Could you check a few things on this model? Use its own coordinates, in mm. Give positions to 0.01 mm unless a question says otherwise; leave off trailing zeros. Write each loop counter-clockwise with the first axis right and the second up, starting at its lowest first coordinate (ties: lowest second). Pieces come first, ordered by that corner, then holes. Notation, with made-up numbers: M 78.25,33 L 85.25,33 A27 ccw 85.25,67 Z; hole C -7.75,7.25 d4. An arc over 180 degrees is marked long. Answer as CSV lines item,"result". Start each with the question number.
from build123d import *

# Parameters (mm, degrees)
SKETCH1_W           = 42.637682839
SKETCH1_H           = 10
BOSS_EXTRUDE1_DEPTH = 2


with BuildPart() as part:
    # Sketch1 → Boss-Extrude1 (new body)
    with BuildSketch(Plane.XY):
        Polygon((0, 20), (9.5, 20), (9.5, 5.999528404), (41.549837727, 5.999528404), (41.549837727, 20), (41.549837727, 22), (80.459837727, 22), (80.459837727, 20), (115.41, 20), (115.41, 15), (117.41, 15), (117.41, 5), (115.41, 5), (115.41, 0), (80.459837727, 0), (80.459837727, -2.000471596), (35.049837727, -2.000471596), (35.049837727, 0), (0, 0), (0, 5), (-2, 5), (-2, 15), (0, 15), align=None)
        with Locations((65.091158581, 11)):
            Rectangle(SKETCH1_W, SKETCH1_H, mode=Mode.SUBTRACT)
    extrude(amount=BOSS_EXTRUDE1_DEPTH)


solid = part.part
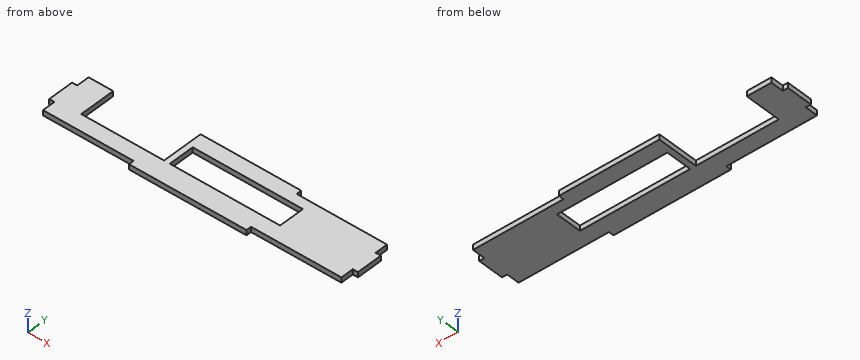
1. Imagine slicing it at B-B, the plane z = 1.1. Please give me the cut outline in (x, y), plus the area to 3 significant figures.
2. Imagine slicing it at A-A, the plane y = 9.5. Please give me the cut outline in (x, z).
3. Imagine slicing it at D-D, the plane y = 18.5. Please give me the cut outline in (x, z).
4. Please list where these lines run through material, in increasing order: line 1 (X direction, y = 11, z = 0.35); line 2 (Y direction, x = 76.5, z = 1.3); line 3 (X direction, y = 16.25, z = 0.6).
5. Imagine slicing it at C-C, the plane x = 75. Please give me the cut outline in (y, z).
6. Will these pins go through, and if not, where does the flat tip stop? P1, Ø1, axis at y = 1, z = 0.5, coming from the +X side; P2, Ø1, axis at x = -1, z = 1, coming from the -Y side; P3, Ø1, axis at x = 101.5, z = 1.5, coming from the +Y side.
Solutions:
1,outline,"M -2,5 L 0,5 L 0,0 L 35.05,0 L 35.05,-2 L 80.46,-2 L 80.46,0 L 115.41,0 L 115.41,5 L 117.41,5 L 117.41,15 L 115.41,15 L 115.41,20 L 80.46,20 L 80.46,22 L 41.55,22 L 41.55,6 L 9.5,6 L 9.5,20 L 0,20 L 0,15 L -2,15 Z; hole M 43.77,6 L 86.41,6 L 86.41,16 L 43.77,16 Z"
1,area,"1,640 mm²"
2,outline,"M -2,0 L 9.5,0 L 9.5,2 L -2,2 Z; M 41.55,0 L 43.77,0 L 43.77,2 L 41.55,2 Z; M 86.41,0 L 117.41,0 L 117.41,2 L 86.41,2 Z"
3,outline,"M 0,0 L 9.5,0 L 9.5,2 L 0,2 Z; M 41.55,0 L 115.41,0 L 115.41,2 L 41.55,2 Z"
4,line 1,"-2 to 9.5, 41.55 to 43.77, 86.41 to 117.41"
4,line 2,"-2 to 6, 16 to 22"
4,line 3,"0 to 9.5, 41.55 to 115.41"
5,outline,"M -2,0 L 6,0 L 6,2 L -2,2 Z; M 16,0 L 22,0 L 22,2 L 16,2 Z"
6,P1,"x = 115.41"
6,P2,"y = 5"
6,P3,"y = 20"
